Geometry check sheet. Reference: the model listing, model coordinates, mm. A direction names the side the tool comes from. Coordinates: 2 decimals unless noted, no trailing zeros. Loops run counter-clockwise (first coordinate to the right, second up) from the corner with the lowest first, then second, coordinate; pieces in that order, holes last. Notation, with made-up numbers: M 45,-11.5 L 81,-11.5 A30 ccw 81,25.5 Z; hole C -12,58.25 d3. An arc over 180 degrees is marked long. Use CSV: the item, a comma, the result in double quotes.
```python
from build123d import *

# Parameters (mm, degrees)
SKETCH1_W           = 50
SKETCH1_H           = 50
BOSS_EXTRUDE1_DEPTH = 12
SKETCH2_R           = 5
CUT_EXTRUDE1_DEPTH  = 58.175169436
CUT_EXTRUDE2_START  = -12.75
SKETCH3_R           = 7.5
CUT_EXTRUDE2_DEPTH  = 24.5
SKETCH4_R           = 2.25
CUT_EXTRUDE3_DEPTH  = 38.336309405
SKETCH5_R           = 4
CUT_EXTRUDE4_DEPTH  = 38.336309405
BOSS_EXTRUDE3_DEPTH = 12
CUT_EXTRUDE5_START  = -15
CUT_EXTRUDE5_DEPTH  = 73.175169436
SKETCH7_W           = 7
SKETCH7_H           = 5
CUT_EXTRUDE6_DEPTH  = 45.068838197
SKETCH13_W          = 10
SKETCH13_H          = 7.25
BOSS_EXTRUDE4_DEPTH = 2
SKETCH14_W          = 14
SKETCH14_H          = 5
BOSS_EXTRUDE5_DEPTH = 10
SKETCH8_W           = 16
SKETCH8_H           = 11
BOSS_EXTRUDE2_DEPTH = 8
CUT_EXTRUDE7_DEPTH  = 15
SKETCH10_W          = 4
SKETCH10_H          = 7
CUT_EXTRUDE8_DEPTH  = 7
CUT_EXTRUDE9_DEPTH  = 4
SKETCH15_W          = 7
SKETCH15_H          = 5
CUT_EXTRUDE10_DEPTH = 46.321766294
BOSS_EXTRUDE6_DEPTH = 12
CUT_EXTRUDE11_REACH = 80.11
SKETCH18_W          = 10
SKETCH18_H          = 18.25
CUT_EXTRUDE12_DEPTH = 59.975100678


with BuildPart() as part:
    # Sketch1 → Boss-Extrude1 (new body)
    with BuildSketch(Plane.XY):
        Rectangle(SKETCH1_W, SKETCH1_H)
    extrude(amount=BOSS_EXTRUDE1_DEPTH)

    # Sketch2 → Cut-Extrude1 (cut, through all)
    with BuildSketch(Plane.ZY.offset(25)):
        with Locations((12, 0)):
            Circle(SKETCH2_R)
    extrude(amount=-CUT_EXTRUDE1_DEPTH, mode=Mode.SUBTRACT)

    # Sketch3 → Cut-Extrude2 (cut)
    with BuildSketch(Plane.ZY.offset(25).offset(CUT_EXTRUDE2_START)):
        with Locations((12, 0)):
            Circle(SKETCH3_R)
    extrude(amount=-CUT_EXTRUDE2_DEPTH, mode=Mode.SUBTRACT)

    # Sketch4 → Cut-Extrude3 (cut, through all)
    with BuildSketch(Plane.XY.offset(12)):
        with Locations((0, 11)):
            Circle(SKETCH4_R)
        with Locations((0, -11)):
            Circle(SKETCH4_R)
    extrude(amount=-CUT_EXTRUDE3_DEPTH, mode=Mode.SUBTRACT)

    # Sketch5 → Cut-Extrude4 (cut, through all)
    with BuildSketch(Plane.XY.offset(12)):
        with Locations((0, 25)):
            Circle(SKETCH5_R)
        with Locations((0, -25)):
            Circle(SKETCH5_R)
    extrude(amount=-CUT_EXTRUDE4_DEPTH, mode=Mode.SUBTRACT)

    # Sketch11 → Boss-Extrude3 (add)
    with BuildSketch(Plane.XY.offset(12)):
        with BuildLine():
            Line((3.464101615, 27), (14, 27))
            Line((14, 27), (14, 34.25))
            Line((14, 34.25), (0, 34.25))
            ThreePointArc((0, 34.25), (-6.540737726, 31.540737726), (-9.25, 25))
            Line((-9.25, 25), (-4, 25))
            ThreePointArc((-4, 25), (-1.03527618, 28.863703305), (3.464101615, 27))
        make_face()
    boss_extrude3 = extrude(amount=-BOSS_EXTRUDE3_DEPTH)

    # Sketch6 → Cut-Extrude5 (cut)
    with BuildSketch(Plane(origin=(0, 25, 0), x_dir=(1, 0, 0), z_dir=(0, 1, 0)).offset(CUT_EXTRUDE5_START)):
        with BuildLine():
            Line((6.409009742, -7.590990258), (8, -9.181980515))
            Line((8, -9.181980515), (9.590990258, -7.590990258))
            ThreePointArc((9.590990258, -7.590990258), (8, -3.75), (6.409009742, -7.590990258))
        make_face()
    cut_extrude5 = extrude(amount=CUT_EXTRUDE5_DEPTH, mode=Mode.SUBTRACT)

    # Sketch7 → Cut-Extrude6 (cut, through all)
    with BuildSketch(Plane.XY.offset(12)):
        with Locations((8, 17.5)):
            Rectangle(SKETCH7_W, SKETCH7_H)
    cut_extrude6 = extrude(amount=-CUT_EXTRUDE6_DEPTH, mode=Mode.SUBTRACT)

    # Sketch13 → Boss-Extrude4 (add)
    with BuildSketch(Plane.XY.offset(12)):
        with Locations((9, 30.625)):
            Rectangle(SKETCH13_W, SKETCH13_H)
    boss_extrude4 = extrude(amount=BOSS_EXTRUDE4_DEPTH)

    # Sketch14 → Boss-Extrude5 (add)
    with BuildSketch(Plane.XY.offset(12)):
        with Locations((7, 31.75)):
            Rectangle(SKETCH14_W, SKETCH14_H)
    boss_extrude5 = extrude(amount=BOSS_EXTRUDE5_DEPTH)

    # Mirror1: Boss-Extrude3, Cut-Extrude5, Cut-Extrude6, Boss-Extrude4, Boss-Extrude5 across plane
    add(boss_extrude3.mirror(Plane.ZX))
    add(cut_extrude5.mirror(Plane.ZX), mode=Mode.SUBTRACT)
    add(cut_extrude6.mirror(Plane.ZX), mode=Mode.SUBTRACT)
    add(boss_extrude4.mirror(Plane.ZX))
    add(boss_extrude5.mirror(Plane.ZX))

    # Sketch8 → Boss-Extrude2 (add)
    with BuildSketch(Plane.ZY.offset(25)):
        with Locations((20, -10.5)):
            Rectangle(SKETCH8_W, SKETCH8_H)
    boss_extrude2 = extrude(amount=-BOSS_EXTRUDE2_DEPTH)

    # Sketch9 → Cut-Extrude7 (cut)
    with BuildSketch(Plane.ZY.offset(25)):
        with BuildLine():
            Line((11.590990258, -8.909009742), (13.181980515, -10.5))
            Line((13.181980515, -10.5), (11.590990258, -12.090990258))
            ThreePointArc((11.590990258, -12.090990258), (7.75, -10.5), (11.590990258, -8.909009742))
        make_face()
        with BuildLine():
            Line((24.590990258, -8.909009742), (26.181980515, -10.5))
            Line((26.181980515, -10.5), (24.590990258, -12.090990258))
            ThreePointArc((24.590990258, -12.090990258), (20.75, -10.5), (24.590990258, -8.909009742))
        make_face()
    cut_extrude7 = extrude(amount=-CUT_EXTRUDE7_DEPTH, mode=Mode.SUBTRACT)

    # Sketch10 → Cut-Extrude8 (cut)
    with BuildSketch(Plane.XY.offset(12)):
        with Locations((-15, -10.5)):
            Rectangle(SKETCH10_W, SKETCH10_H)
    cut_extrude8 = extrude(amount=-CUT_EXTRUDE8_DEPTH, mode=Mode.SUBTRACT)

    # Mirror2: Boss-Extrude2, Cut-Extrude7, Cut-Extrude8 across plane
    add(boss_extrude2.mirror(Plane(origin=(0, 0, 0), x_dir=(0, 0, 1), z_dir=(1, 0, 0))))
    add(cut_extrude7.mirror(Plane(origin=(0, 0, 0), x_dir=(0, 0, 1), z_dir=(1, 0, 0))), mode=Mode.SUBTRACT)
    add(cut_extrude8.mirror(Plane(origin=(0, 0, 0), x_dir=(0, 0, 1), z_dir=(1, 0, 0))), mode=Mode.SUBTRACT)

    # Sketch12 → Cut-Extrude9 (cut)
    with BuildSketch(Plane(origin=(0, -34.25, 0), x_dir=(1, 0, 0), z_dir=(0, 1, 0))):
        with BuildLine():
            Line((5.171572875, -8.828427125), (8, -11.656854249))
            Line((8, -11.656854249), (10.828427125, -8.828427125))
            ThreePointArc((10.828427125, -8.828427125), (8, -2), (5.171572875, -8.828427125))
        make_face()
    extrude(amount=CUT_EXTRUDE9_DEPTH, mode=Mode.SUBTRACT)

    # Sketch15 → Cut-Extrude10 (cut, through all)
    with BuildSketch(Plane.XY.offset(12)):
        with Locations((-8, 17.5)):
            Rectangle(SKETCH15_W, SKETCH15_H)
    extrude(amount=-CUT_EXTRUDE10_DEPTH, mode=Mode.SUBTRACT)

    # Sketch16 → Boss-Extrude6 (add)
    with BuildSketch(Plane.XY.offset(12)):
        with BuildLine():
            Line((-14, 25), (-4, 25))
            ThreePointArc((-4, 25), (-2.828427125, 27.828427125), (0, 29))
            Line((0, 29), (0, 34.25))
            Line((0, 34.25), (-14, 34.25))
            Line((-14, 34.25), (-14, 25))
        make_face()
    extrude(amount=-BOSS_EXTRUDE6_DEPTH)

    # Cut-Extrude11: up to this face of the body (flat: up to its plane)
    cut_extrude11_end = Plane(part.part.faces().sort_by_distance((8, 10, 6.158015302))[0])
    # Sketch17 → Cut-Extrude11 (cut, up to the picked face)
    with BuildSketch(Plane(origin=(0, 34.25, 0), x_dir=(1, 0, 0), z_dir=(0, 1, 0)), mode=Mode.PRIVATE) as cut_extrude11_sk1:
        with BuildLine():
            Line((-9.590990258, -7.590990258), (-8, -9.181980515))
            Line((-8, -9.181980515), (-6.409009742, -7.590990258))
            ThreePointArc((-6.409009742, -7.590990258), (-8, -3.75), (-9.590990258, -7.590990258))
        make_face()
    cut_extrude11_tool1 = split(extrude(cut_extrude11_sk1.sketch, amount=-CUT_EXTRUDE11_REACH, mode=Mode.PRIVATE), bisect_by=cut_extrude11_end, keep=Keep.BOTH, mode=Mode.PRIVATE)
    add(cut_extrude11_tool1.solids().sort_by(Axis((-8, 34.25, 6.158015), (0, -1, 0)))[0], mode=Mode.SUBTRACT)

    # Sketch18 → Cut-Extrude12 (cut, through all)
    with BuildSketch(Plane(origin=(14, 0, 0), x_dir=(0, 0, -1), z_dir=(1, 0, 0))):
        with Locations((-17, -25.125)):
            Rectangle(SKETCH18_W, SKETCH18_H)
    extrude(amount=-CUT_EXTRUDE12_DEPTH, mode=Mode.SUBTRACT)


solid = part.part
```
1. Section check A-A, the plane y = -28. Record the cut outline in (x, z), plus the area to 3 significant figures.
The answers:
outline,"M -8.75,0 L -2.65,0 L -2.65,12 L -8.75,12 Z; M 2.65,0 L 14,0 L 14,12 L 2.65,12 Z; hole M 6.41,7.59 A2.25 ccw long 9.59,7.59 L 8,9.18 Z"
area,"193 mm^2"
2. Section check B-B, the plane x = -18.5. Record the cut outline in (y, z).
The answers:
outline,"M -25,0 L 25,0 L 25,12 L 5,12 A5 cw -5,12 L -5,28 L -16,28 L -16,12 L -25,12 Z; hole M -12.09,11.59 A2.25 ccw long -8.91,11.59 L -10.5,13.18 Z; hole M -12.09,24.59 A2.25 ccw long -8.91,24.59 L -10.5,26.18 Z"
3. Release check for a two-part mould opening along Y. For faces 5 (the flat face through (-10.4, 20, 6.1)), 6 (the cylindrical face through (8.07, -28.6, 3.75)) record: +Y half, -Y half, draft (parallel to the pull), parting line (faces both ways), or undercut.
The answers:
face 5,"undercut"
face 6,"draft"
4. Set-up check for faces 1 (the cylindrical face through (8.07, 22.46, 3.75)), 2 (the flat face through (5.6, 15, 6.1)), 3 (the flat face through (8.78, -28.6, 8.4)), 4 (the flat face through (10, 27, 8)): record each of +Z, -Z, +X, -X, +Y, -Y from which the full face is reachable in a straight line by a thin tool's end or side.
The answers:
face 1,"+Y"
face 2,"+Z, -Z"
face 3,"-Y"
face 4,"+Z, -Z, +X"
5. Section check C-C, the plane z = 23. Record the cut outline in (x, y), plus the area to 3 significant figures.
The answers:
outline,"M -25,-16 L -17,-16 L -17,-12.75 L -25,-12.75 Z; M -25,-8.25 L -17,-8.25 L -17,-5 L -25,-5 Z; M 17,-16 L 25,-16 L 25,-12.75 L 17,-12.75 Z; M 17,-8.25 L 25,-8.25 L 25,-5 L 17,-5 Z"
area,"104 mm^2"
6. Section check D-D, the plane x = 1. Record the cut outline in (y, z), plus the area to 3 significant figures.
The answers:
outline,"M -34.25,0 L -28.87,0 L -28.87,12 L -34.25,12 Z; M -21.13,0 L -13.02,0 L -13.02,12 L -21.13,12 Z; M -8.98,0 L 8.98,0 L 8.98,12 L 7.5,12 A7.5 cw -7.5,12 L -8.98,12 Z; M 13.02,0 L 21.13,0 L 21.13,12 L 13.02,12 Z; M 28.87,0 L 34.25,0 L 34.25,22 L 29.25,22 L 29.25,12 L 28.87,12 Z"
area,"501 mm^2"
7. Gauge pin test, flat ends, axial feed: P1, Ø1.4, axis at x = 7.5, z = 6.5, coming from the -Y side; P2, Ø4, axis at x = 8, z = 6, coming from the +Y side; P3, Ø5.5, axis at x = -17.5, z = 5, coming from the +Y side. Record the tip position at first contact, or that the pin passes through.
The answers:
P1,"y = -10"
P2,"y = 10"
P3,"y = 25"
8. Thickness scan on line 1 (X direction, y = 32.5, z = 6); line 2 (X direction, y = 13.85, z = 6); line 3 (Y direction, x = 0, z = 3.75). Record the ranges inside material, lowest first. Write a range as [from, to].
The answers:
line 1,"[-14, -10.25], [-5.75, 5.75], [10.25, 14]"
line 2,"[-25, -10.25], [-5.75, 5.75], [10.25, 25]"
line 3,"[-34.25, -29], [-21, -13.25], [-8.75, 8.75], [13.25, 21], [29, 34.25]"
